Model file for the job. Use its own axes, mm. Round coordinates to 2 decimals unless told otherwise and drop trailing zeros. Write each loop counter-clockwise with the first axis right and the second up, starting at its lowest first coordinate (ties: lowest second). Pieces come first, ordered by that corner, then holes.
```python
from build123d import *

# Parameters (mm, degrees)
SKETCH1_W           = 200
SKETCH1_H           = 100
BOSS_EXTRUDE1_DEPTH = 4.15
SKETCH3_W           = 19.52
SKETCH3_H           = 3.91
CUT_EXTRUDE2_DEPTH  = 10
SKETCH4_W           = 3.91
SKETCH4_H           = 19.52
CUT_EXTRUDE3_DEPTH  = 10
SKETCH21_W          = 3
SKETCH21_H          = 5
CUT_EXTRUDE22_DEPTH = 4.2


with BuildPart() as part:
    # Sketch1 → Boss-Extrude1 (new body)
    with BuildSketch(Plane(origin=(0, 0, 0), x_dir=(1, 0, 0), z_dir=(0, 1, 0))):
        Rectangle(SKETCH1_W, SKETCH1_H)
    extrude(amount=BOSS_EXTRUDE1_DEPTH)

    # Sketch3 → Cut-Extrude2 (cut)
    with BuildSketch(Plane(origin=(0, 4.15, 0), x_dir=(1, 0, 0), z_dir=(0, 1, 0))):
        with Locations((-90.24, 48.045)):
            Rectangle(SKETCH3_W, SKETCH3_H)
        with Locations((-90.24, -48.045)):
            Rectangle(SKETCH3_W, SKETCH3_H)
        with Locations((-50.24, 48.045)):
            Rectangle(SKETCH3_W, SKETCH3_H)
        with Locations((-10.24, 48.045)):
            Rectangle(SKETCH3_W, SKETCH3_H)
        with Locations((29.76, 48.045)):
            Rectangle(SKETCH3_W, SKETCH3_H)
        with Locations((69.76, 48.045)):
            Rectangle(SKETCH3_W, SKETCH3_H)
        with Locations((-50.24, -48.045)):
            Rectangle(SKETCH3_W, SKETCH3_H)
        with Locations((-10.24, -48.045)):
            Rectangle(SKETCH3_W, SKETCH3_H)
        with Locations((29.76, -48.045)):
            Rectangle(SKETCH3_W, SKETCH3_H)
        with Locations((69.76, -48.045)):
            Rectangle(SKETCH3_W, SKETCH3_H)
    extrude(amount=-CUT_EXTRUDE2_DEPTH, mode=Mode.SUBTRACT)

    # Sketch4 → Cut-Extrude3 (cut)
    with BuildSketch(Plane(origin=(0, 4.15, 0), x_dir=(1, 0, 0), z_dir=(0, 1, 0))):
        with Locations((-98.045, 0)):
            Rectangle(SKETCH4_W, SKETCH4_H)
        with Locations((98.045, 0)):
            Rectangle(SKETCH4_W, SKETCH4_H)
    extrude(amount=-CUT_EXTRUDE3_DEPTH, mode=Mode.SUBTRACT)

    # Sketch21 → Cut-Extrude22 (cut)
    with BuildSketch(Plane(origin=(0, 4.15, 0), x_dir=(1, 0, 0), z_dir=(0, 1, 0))):
        with Locations((23.31, 23.41)):
            Rectangle(SKETCH21_W, SKETCH21_H)
    extrude(amount=-CUT_EXTRUDE22_DEPTH, mode=Mode.SUBTRACT)


solid = part.part
```
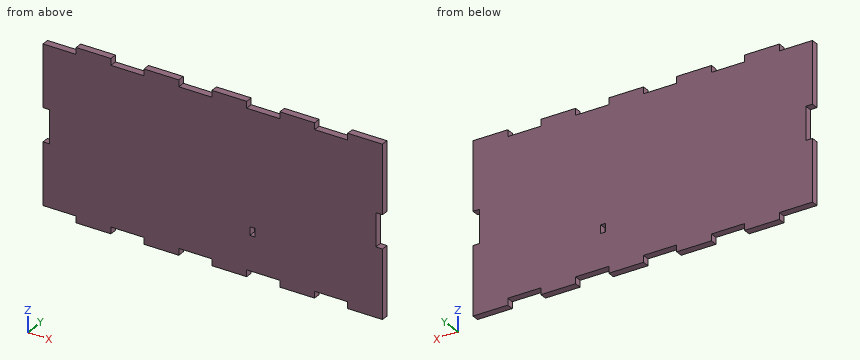
1) Cut at A-A on x = -6. List the corners of the cut face in (y, z), and give its area (3 significant figures).
2) Flat gauge pins, fed straight in: pin 1 Ø1.2 at (y, z) = (1.5, -47.5) entering from -X; pin 2 Ø1.2 at (y, z) = (2.5, -1) entering from +X; pin 3 Ø1 at (x, y) = (-12, 2) entering from +Z. Where does each tip first touch, or does it go through?
3) Wall check: probe 1 along X at (y, z) = (3.4, -25.5); probe 2 along Z at (x, y) = (79, 1.1); probe 3 along X at (y, z) = (1.35, 8). Give the ranges that are in metal, low to high.
4) Cut at B-B on z = -5. List the corners of the cut face in (x, y), and give its area (3 significant figures).
Result sheet:
1. outline: (0, -46.09) - (4.15, -46.09) - (4.15, 46.09) - (0, 46.09) - close
1. area: 383 mm2
2. pin 1: stops at x = -80.48
2. pin 2: stops at x = 96.09
2. pin 3: stops at z = 46.09
3. probe 1: x = -100 to 21.81, 24.81 to 100
3. probe 2: z = -46.09 to 46.09
3. probe 3: x = -96.09 to 96.09
4. outline: (-96.09, 0) - (96.09, 0) - (96.09, 4.15) - (-96.09, 4.15) - close
4. area: 798 mm2
